from build123d import *

# Parameters (mm, degrees)
BOSS_EXTRUDE1_DEPTH = 3.175
FILLET1_R           = 80
FILLET2_R           = 8
SKETCH2_R           = 1.65
CUT_EXTRUDE1_DEPTH  = 10


with BuildPart() as part:
    # Sketch1 → Boss-Extrude1 (new body)
    with BuildSketch(Plane(origin=(0, 0, 0), x_dir=(1, 0, 0), z_dir=(0, 1, 0))):
        with BuildLine():
            Line((-70, 14), (-40, 14))
            Line((-40, 14), (-39.816062711, 70))
            Line((-39.816062711, 70), (-73.623466631, 79.058666579))
            ThreePointArc((-73.623466631, 79.058666579), (-83.522961568, 96.205094778), (-66.376533369, 106.104589715))
            Line((-66.376533369, 106.104589715), (0, 88.319051202))
            Line((0, 88.319051202), (66.376533369, 106.104589715))
            ThreePointArc((66.376533369, 106.104589715), (83.522961568, 96.205094778), (73.623466631, 79.058666579))
            Line((73.623466631, 79.058666579), (39.816062711, 70))
            Line((39.816062711, 70), (40, 14))
            Line((40, 14), (70, 14))
            ThreePointArc((70, 14), (84, 0), (70, -14))
            Line((70, -14), (40, -14))
            Line((40, -14), (39.816062711, -70))
            Line((39.816062711, -70), (73.623466631, -79.058666579))
            ThreePointArc((73.623466631, -79.058666579), (83.522961568, -96.205094778), (66.376533369, -106.104589715))
            Line((66.376533369, -106.104589715), (0, -88.319051202))
            Line((0, -88.319051202), (-66.376533369, -106.104589715))
            ThreePointArc((-66.376533369, -106.104589715), (-83.522961568, -96.205094778), (-73.623466631, -79.058666579))
            Line((-73.623466631, -79.058666579), (-39.816062711, -70))
            Line((-39.816062711, -70), (-40, -14))
            Line((-40, -14), (-70, -14))
            ThreePointArc((-70, -14), (-84, 0), (-70, 14))
        make_face()
    extrude(amount=BOSS_EXTRUDE1_DEPTH)

    # Fillet1
    fillet1_edges = [part.edges().sort_by_distance(p)[0] for p in [
        (0, 1.5875, -88.319051202),
        (0, 1.5875, 88.319051202),
    ]]
    fillet(fillet1_edges, radius=FILLET1_R)

    # Fillet2
    fillet2_edges = [part.edges().sort_by_distance(p)[0] for p in [
        (-40, 1.5875, -14),
        (-39.816062711, 1.5875, -70),
        (39.816062711, 1.5875, -70),
        (40, 1.5875, -14),
        (40, 1.5875, 14),
        (39.816062711, 1.5875, 70),
        (-39.816062711, 1.5875, 70),
        (-40, 1.5875, 14),
    ]]
    fillet(fillet2_edges, radius=FILLET2_R)

    # Sketch2 → Cut-Extrude1 (cut)
    with BuildSketch(Plane(origin=(0, 3.175, 0), x_dir=(1, 0, 0), z_dir=(0, 1, 0))):
        with Locations(Location((0, 87.141145635, 0), (0, 0, 270))):
            Circle(SKETCH2_R)
        with Locations(Location((-35.905030257, 42.907120147, 0), (0, 0, 270))):
            Circle(SKETCH2_R)
        with Locations(Location((35.905030257, 42.907120147, 0), (0, 0, 270))):
            Circle(SKETCH2_R)
        with Locations(Location((35.905030257, -42.907120147, 0), (0, 0, 270))):
            Circle(SKETCH2_R)
        with Locations(Location((0, -87.141145635, 0), (0, 0, 270))):
            Circle(SKETCH2_R)
        with Locations(Location((-35.905030257, -42.907120147, 0), (0, 0, 270))):
            Circle(SKETCH2_R)
    extrude(amount=-CUT_EXTRUDE1_DEPTH, mode=Mode.SUBTRACT)


solid = part.part
Geometry: final body of the model. Coordinates: model frame, mm. A direction names the side the tool comes from. Coordinates: 2 decimals unless noted, no trailing zeros. Loops run counter-clockwise (first coordinate to the right, second up) from the corner with the lowest first, then second, coordinate; pieces in that order, holes last. Notation, with made-up numbers: (-37.75, 1.25) - (-10.75, 1.25) arc R22 ccw to (-10.75, 36.25) - close; hole circle Ø4 at (45, -4.75). An arc over 180 degrees is marked (long way). Put each result on its own line as item: value. Start each with the question number.
Q1. Pin query (flat end, axial travel): pin 1 Ø1 at (x, y) = (-62, 2) entering from -Z. Return the tip coordinate at first contact, or that it passes through.
Q2. Cut plane B-B, the plane x = 26. Return loops of the section in (y, z) (3 decimals), and give its area (3 significant figures).
Q3. Pull-direction query (Z, two-part tool) for faces 1 (the flat face through (-59.89, 1.57, 75.38)), 2 (the flat face through (1, 0, -1)), 3 (the flat face through (-43.86, 1.57, -100.07)), 4 (the flat face through (59.89, 1.57, -75.38)); classes: released by +Z, released by -Z, zero draft, split by the parting line, or undercut.
Q4. Line query: line 1 (Z direction, x = 59.5, y = 0.35); line 2 (Z direction, x = 71, y = 1.6); line 3 (X direction, y = 1.1, z = -36). Output: solid intervals per line, ascending.
Q5. Set-up query: faces 5 (the cylindrical face through (-42.39, 1.61, 16.27)), 6 (the flat face through (43.22, 1.57, -99.9)), 7 (the flat face through (59.5, 1.565, 75.274)), 8 (the flat face through (43.86, 1.57, 100.07)). Return all of +Z, -Z, +X, -X, +Y, -Y with unobstructed straight access to the full face (end or side cutting, diameter ignored); none if empty.
Q6. Cut plane A-A, the plane z = 25. Return loops of the section in (x, y) (3 decimals).
Filled sheet:
1. pin 1: z = -105.07
2. outline: (0, -95.286) - (3.175, -95.286) - (3.175, 95.286) - (0, 95.286) - close
2. area: 605 mm²
3. face 1: undercut
3. face 2: zero draft
3. face 3: released by -Z
3. face 4: undercut
4. line 1: -104.26 to -75.27, -14 to 14, 75.27 to 104.26
4. line 2: -106.55 to -78.36, -13.96 to 13.96, 78.36 to 106.55
4. line 3: -39.93 to 39.93
5. face 5: -X, +Y, -Y
5. face 6: -Z, +Y, -Y
5. face 7: +X, +Y, -Y
5. face 8: +Z, +Y, -Y
6. outline: (-39.964, 0) - (39.964, 0) - (39.964, 3.175) - (-39.964, 3.175) - close
